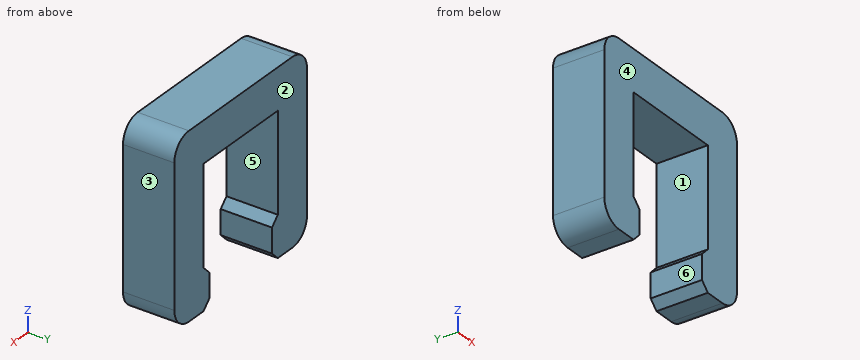
from build123d import *

# Parameters (mm, degrees)
BOSS_EXTRUDE1_DEPTH = 3.175
FILLET1_R           = 1.27


with BuildPart() as part:
    # Sketch1 → Boss-Extrude1 (new body)
    with BuildSketch(Plane(origin=(0, 0, 0), x_dir=(1, 0, 0), z_dir=(0, 1, 0))):
        Polygon((-5.7785, 5.588), (-5.7785, -5.588), (5.7785, -5.588), (5.7785, 5.588), (3.2385, 5.588), (2.7305, 5.08), (2.7305, 3.556), (3.2385, 3.048), (3.2385, -3.048), (-3.2385, -3.048), (-3.2385, 3.048), (-2.7305, 3.556), (-2.7305, 5.08), (-3.2385, 5.588), align=None)
    extrude(amount=BOSS_EXTRUDE1_DEPTH)

    # Fillet1
    fillet1_edges = [part.edges().sort_by_distance(p)[0] for p in [
        (5.7785, 1.5875, -5.588),
        (5.7785, 1.5875, 5.588),
        (-5.7785, 1.5875, 5.588),
        (-5.7785, 1.5875, -5.588),
    ]]
    fillet(fillet1_edges, radius=FILLET1_R)


solid = part.part
Source: CAD feature listing. Evaluate the final solid. Frame: model axes, mm. Face numbers are marked on the shaded views. A direction names the side the tool comes from. Round coordinates to 2 decimals unless told otherwise and drop trailing zeros. Loops run counter-clockwise (first coordinate to the right, second up) from the corner with the lowest first, then second, coordinate; pieces in that order, holes last. Notation, with made-up numbers: M 8.25,-35 L 40.25,-35 A18 cw 40.25,-11 Z; hole C -26.5,-12.75 d6. An arc over 180 degrees is marked long. Return JSON: item names as keys, results as strings. Group by question number.
1. Section query D-D on x = 0. Output: boundary loops of the cut face in (y, z) (3 decimals), and give its area (3 significant figures).
2. Section query C-C on y = 2.1. Output: boundary loops of the cut face in (x, z), and give its area (3 significant figures).
3. Pin query (flat end, axial travel): pin 1 (1 mm diameter, centred on x = 1, y = 2, fed in from -Z). Return the tip coordinate at first contact, or that it passes through.
4. Section query A-A on z = 2.5. Output: boundary loops of the cut face in (x, y) (1 decimal).
5. Material intervals for line 1 along X through (y, z) = (1.85, 2.5); line 2 along Z through (x, y) = (-1.75, 0.2); line 3 along Z through (x, y) = (-3, 1.75), sorted ascending. Write a range as from..to.
6. Section query B-B on x = 3. Output: boundary loops of the cut face in (y, z) (1 decimal), and give its area (3 significant figures).
7. Reachability of the marked faces 1 and 2 from +Z, -Z, +X, -X, +Y, -Y: full face, straight path, thin tool, end or side. Return the list, or none.
8. Mould query, pull axis X, two halves, no side actions, for the marked faces 3, 4, 5 and 6. Classes: released by +X, released by -X, zero draft, split by the parting line, or undercut.
Checks:
{
 "1": {"outline": "M 0,3.048 L 3.175,3.048 L 3.175,5.588 L 0,5.588 Z", "area": "8.06 mm²"},
 "2": {"outline": "M -5.78,-4.32 A1.27 ccw -4.51,-5.59 L -3.24,-5.59 L -2.73,-5.08 L -2.73,-3.56 L -3.24,-3.05 L -3.24,3.05 L 3.24,3.05 L 3.24,-3.05 L 2.73,-3.56 L 2.73,-5.08 L 3.24,-5.59 L 4.51,-5.59 A1.27 ccw 5.78,-4.32 L 5.78,4.32 A1.27 ccw 4.51,5.59 L -4.51,5.59 A1.27 ccw -5.78,4.32 Z", "area": "73.9 mm²"},
 "3": {"pin 1": "stops at z = 3.05"},
 "4": {"outline": "M -5.8,0 L -3.2,0 L -3.2,3.2 L -5.8,3.2 Z; M 3.2,0 L 5.8,0 L 5.8,3.2 L 3.2,3.2 Z"},
 "5": {"line 1": "x = -5.78..-3.24, 3.24..5.78", "line 2": "z = 3.05..5.59", "line 3": "z = -5.35..-3.29, 3.05..5.59"},
 "6": {"outline": "M 0,-5.3 L 3.2,-5.3 L 3.2,-3.3 L 0,-3.3 Z; M 0,3 L 3.2,3 L 3.2,5.6 L 0,5.6 Z", "area": "14.6 mm²"},
 "7": {"face 1": "+Y, -Y", "face 2": "+Z, -Z, +X, -X, +Y"},
 "8": {"face 3": "released by +X", "face 4": "zero draft", "face 5": "undercut", "face 6": "undercut"}
}
